Can you work these out from the drawing? Everything is in mm from the part's minimum corner. A direction names the side the tool comes from. Round coordinates to 2 decimals unless told otherwise and drop trailing zeros. Loops run counter-clockwise (first coordinate to the right, second up) from the corner with the lowest first, then second, coordinate; pieces in that order, holes last. Notation, with made-up numbers: M -11,14 L -5,14 A13 cw -5,19 Z; hole C 67.25,-24 d9. An arc over 180 degrees is marked long. Use a Markdown table: item, result.
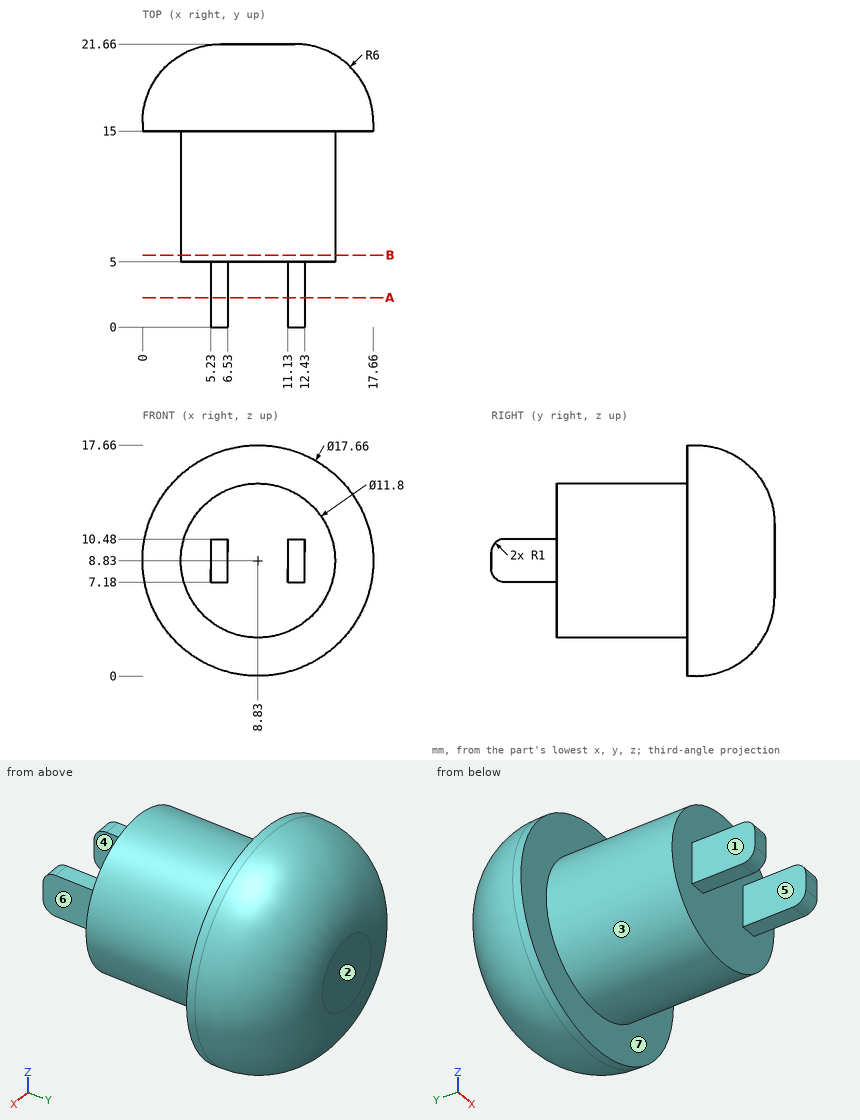
1. For pin 1 Ø6 at (y, z) = (11.5, 3.5) entering from -X; pin 2 Ø1.7 at (y, z) = (3.5, 9) entering from +X; pin 3 Ø4 at (x, y) = (12, 18) entering from -Z; pin 4 Ø9.5 at (x, z) = (9.5, 8.5) entering from -Y, each with a flat end and sliding along its axis, tell me the tip position at first contact or that it passes through.
Answer sheet:
| item | result |
|---|---|
| pin 1 | x = 3.41 |
| pin 2 | x = 12.43 |
| pin 3 | z = 0.25 |
| pin 4 | y = 0 |
2. I need wall thicknesses on probe 1 along Y at (x, z) = (11, 10); probe 2 along Z at (x, y) = (7, 15.5); probe 3 along X at (y, z) = (16.75, 16.75). Which ranges of each line are inside material? Lowest first, please. Write a range as from..to.
Answer sheet:
| item | result |
|---|---|
| probe 1 | 5..21.66 |
| probe 2 | 0.19..17.47 |
| probe 3 | 5.16..12.5 |
3. We'd pull the mould along X, two halves only. Please class the marked faces 4, 5, 6 and 7: +X half, -X half, draft (parallel to the pull), parting line (faces both ways), or undercut.
Answer sheet:
| item | result |
|---|---|
| face 4 | undercut |
| face 5 | undercut |
| face 6 | +X half |
| face 7 | draft |
4. Imagine slicing it at B-B, the plane y = 5.5. Write out the boundary of the cut face in (x, z).
Answer sheet:
| item | result |
|---|---|
| outline | C 8.83,8.83 d11.8 |
5. Imagine slicing it at A-A, the plane y = 2.25. Write out the boundary of the cut face in (x, z).
Answer sheet:
| item | result |
|---|---|
| outline | M 5.23,7.18 L 6.53,7.18 L 6.53,10.48 L 5.23,10.48 Z; M 11.13,7.18 L 12.43,7.18 L 12.43,10.48 L 11.13,10.48 Z |
6. Which directions (+Z, -Z, +X, -X, +Y, -Y) give clear straight access to the entire face, cutting with the end or side of a thin tool? Please do the marked faces 1, 2 and 3.
Answer sheet:
| item | result |
|---|---|
| face 1 | +Z, -Z, -X, -Y |
| face 2 | +Z, -Z, +X, -X, +Y |
| face 3 | -Y |
